The model under review builds one solid part; all positions refer to its coordinate system, in mm. Face numbers are marked on the shaded views. Give positions to 0.01 mm unless a question says otherwise; leave off trailing zeros. Loops run counter-clockwise (first coordinate to the right, second up) from the corner with the lowest first, then second, coordinate; pieces in that order, holes last. Notation, with made-up numbers: M -33.5,19 L -27.5,19 A18 ccw -27.5,25 Z; hole C 26,-27 d10. An arc over 180 degrees is marked long. Write item = value, one per line. Start each with the question number.
1. We need section A-A on z = 0. Give the boundary of the cut face in (x, y), then the cut area to 3 significant figures.
2. Draft analysis for pull direction Y (two halves, no side actions). For the marked faces 1, 2 and 3, state which applies: pulls with the +Y half, pulls with the -Y half, needs draft (parallel to the pull), parting line crosses it, or undercut.
3. We need section B-B on y = 0. Give the boundary of the cut face in (x, z), then the cut area to 3 significant figures.
4. For pin 1 (1.5 mm diameter, centred on y = 33.5, z = -110.5, fed in from -X); pin 2 (2 mm diameter, centred on x = -28.5, y = 8, fed in from -Z); pin 3 (4 mm diameter, centred on x = 34.5, y = 33, fed in from -Z), all flat-tipped, find the tip position at first contact; note any pin that passes through.
5. Wall thickness on line 1 along Y through (x, z) = (27, 0); line 2 along X through (y, z) = (21, -102); line 3 along Y through (x, z) = (-8, -9): over which ranges is each line inside the solid? List them lowest first. Write a range as from..to.
6. We need section D-D on y = 106. Give the boundary of the cut face in (x, z), then the cut area to 3 significant figures.
7. We need section C-C on x = 28. Give the boundary of the cut face in (y, z), then the cut area to 3 significant figures.
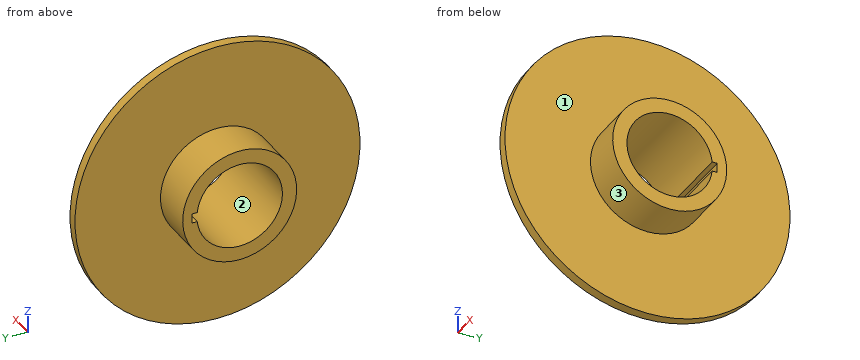
from build123d import *

# Parameters (mm, degrees)
SKETCH1_R           = 60
BOSS_EXTRUDE1_DEPTH = 50
SKETCH1_3_R         = 150
SKETCH1_3_R_2       = 60
BOSS_EXTRUDE2_DEPTH = 5


with BuildPart() as part:
    # Sketch1 → Boss-Extrude1 (new, symmetric)
    with BuildSketch(Plane(origin=(0, 0, 0), x_dir=(0, 0, -1), z_dir=(1, 0, 0))):
        Circle(SKETCH1_R)
        with BuildLine():
            ThreePointArc((45, 0), (-30, -33.541019662), (-5, 44.72135955))
            Line((-5, 44.72135955), (-5, 50))
            Line((-5, 50), (5, 50))
            Line((5, 50), (5, 44.72135955))
            ThreePointArc((5, 44.72135955), (33.541019662, 30), (45, 0))
        make_face(mode=Mode.SUBTRACT)
    extrude(amount=BOSS_EXTRUDE1_DEPTH, both=True)

    # Sketch1<3> → Boss-Extrude2 (add, symmetric)
    with BuildSketch(Plane(origin=(0, 0, 0), x_dir=(0, 0, -1), z_dir=(1, 0, 0))):
        Circle(SKETCH1_3_R)
        Circle(SKETCH1_3_R_2, mode=Mode.SUBTRACT)
    extrude(amount=BOSS_EXTRUDE2_DEPTH, both=True)


solid = part.part
Final values:
q1.outline = M -50,-60 L -5,-60 L -5,-150 L 5,-150 L 5,-60 L 50,-60 L 50,-45 L -50,-45 Z; M -50,50 L 50,50 L 50,60 L 5,60 L 5,150 L -5,150 L -5,60 L -50,60 Z
q1.area = 4,300 mm²
q2.face_1 = needs draft
q2.face_2 = undercut
q2.face_3 = parting line crosses it
q3.outline = M -50,-60 L -5,-60 L -5,-150 L 5,-150 L 5,-60 L 50,-60 L 50,-45 L -50,-45 Z; M -50,45 L 50,45 L 50,60 L 5,60 L 5,150 L -5,150 L -5,60 L -50,60 Z
q3.area = 4,800 mm²
q4.pin_1 = -5
q4.pin_2 = -59.59
q4.pin_3 = -51.37
q5.line_1 = -60..-45, 50..60
q5.line_2 = -5..5
q5.line_3 = -59.32..-44.09, 44.09..59.32
q6.outline = M -5,-106.13 L 5,-106.13 L 5,106.13 L -5,106.13 Z
q6.area = 2,120 mm²
q7.outline = C 0,0 d120; hole M 44.72,-5 L 50,-5 L 50,5 L 44.72,5 A45 ccw long Z
q7.area = 4,900 mm²
